Part model, mm, in its own coordinate system. A direction names the side the tool comes from. Give positions to 0.01 mm unless a question says otherwise; leave off trailing zeros. Loops run counter-clockwise (first coordinate to the right, second up) from the corner with the lowest first, then second, coordinate; pieces in that order, holes last. Notation, with made-up numbers: M 11.25,85.5 L 29.25,85.5 A30 ccw 29.25,109.5 Z; hole C 53,46 d3. An arc over 180 degrees is marked long. Answer in a Markdown table with one row per item.
from build123d import *

# Parameters (mm, degrees)
SKETCH1_W           = 83.5
SKETCH1_H           = 50
BOSS_EXTRUDE1_DEPTH = 1
SKETCH2_W           = 75
SKETCH2_H           = 15
BOSS_EXTRUDE2_DEPTH = 12.8
SKETCH3_W           = 3.3
SKETCH3_H           = 8.9
BOSS_EXTRUDE3_DEPTH = 11
BOSS_EXTRUDE4_DEPTH = 10.3
BOSS_EXTRUDE6_DEPTH = 0.5
BOSS_EXTRUDE7_DEPTH = 0.5
SKETCH7_W           = 2.9
SKETCH7_H           = 2.1
BOSS_EXTRUDE8_DEPTH = 0.8
SKETCH8_R           = 2.25
CUT_EXTRUDE1_DEPTH  = 12.2


with BuildPart() as part:
    # Sketch1 → Boss-Extrude1 (new body)
    with BuildSketch(Plane.XY):
        Rectangle(SKETCH1_W, SKETCH1_H)
    extrude(amount=BOSS_EXTRUDE1_DEPTH)

    # Sketch2 → Boss-Extrude2 (add)
    with BuildSketch(Plane.XY.offset(1)):
        with Locations((2.25, 26)):
            Rectangle(SKETCH2_W, SKETCH2_H)
    extrude(amount=BOSS_EXTRUDE2_DEPTH)



with BuildPart() as body_2:
    # Sketch3 → Boss-Extrude3 (new body)
    with BuildSketch(Plane.XY.offset(1)):
        with Locations((-45.1, -20.15)):
            Rectangle(SKETCH3_W, SKETCH3_H)
    extrude(amount=BOSS_EXTRUDE3_DEPTH)


with BuildPart() as part_1:
    add(part.part)

    add(body_2.part)  # Boss-Extrude4 merges body 2
    # Sketch4 → Boss-Extrude4 (add)
    with BuildSketch(Plane(origin=(-43.45, 0, 0), x_dir=(0, 0, -1), z_dir=(1, 0, 0))):
        with BuildLine():
            Line((-7.3, -16.2), (-1, -16.2))
            Line((-1, -16.2), (-1, -24.1))
            Line((-1, -24.1), (-7.3, -24.1))
            ThreePointArc((-7.3, -24.1), (-11.25, -20.15), (-7.3, -16.2))
        make_face()
    extrude(amount=BOSS_EXTRUDE4_DEPTH)

    # Sketch5 → Boss-Extrude6 (add)
    with BuildSketch(Plane.XZ.offset(24.1)):
        Polygon((-34.55, 7.3), (-34.55, 1), (-41.75, 1), (-43.45, 1), (-43.45, 7.3), align=None)
    extrude(amount=BOSS_EXTRUDE6_DEPTH)

    # Sketch6 → Boss-Extrude7 (add)
    with BuildSketch(Plane(origin=(0, -16.2, 0), x_dir=(1, 0, 0), z_dir=(0, 1, 0))):
        Polygon((-43.45, -7.3), (-34.55, -7.3), (-34.55, -1), (-41.75, -1), (-43.45, -1), align=None)
    extrude(amount=BOSS_EXTRUDE7_DEPTH)

    # Sketch7 → Boss-Extrude8 (add)
    with BuildSketch(Plane(origin=(-33.15, 0, 0), x_dir=(0, 0, -1), z_dir=(1, 0, 0))):
        with Locations((-2.45, -23.05)):
            Rectangle(SKETCH7_W, SKETCH7_H)
        with Locations((-2.45, -17.25)):
            Rectangle(SKETCH7_W, SKETCH7_H)
    extrude(amount=BOSS_EXTRUDE8_DEPTH)

    # Sketch8 → Cut-Extrude1 (cut)
    with BuildSketch(Plane.ZY.offset(46.75)):
        with Locations((7.3, -20.15)):
            Circle(SKETCH8_R)
    extrude(amount=-CUT_EXTRUDE1_DEPTH, mode=Mode.SUBTRACT)


solid = part_1.part
(1) Which spindle directions (+Z, -Z, +X, -X, +Y, -Y) get a long thin tool onto all of the face, cutting with end or side? Do faces 5 (the face through (-34, -16.2, 4)), 6 (the face through (-42, -24.6, 5)), 7 (the face through (2, 29, 1)), 8 (the face through (-35.25, 26, 7)), 9 (the face through (-32.35, -17, 2)). Say none if no direction does.
Recorded:
| item | result |
|---|---|
| face 5 | +Z, +X |
| face 6 | +Z, +X, -X, -Y |
| face 7 | -Z, +X, -X, +Y |
| face 8 | +Z, -X, +Y |
| face 9 | +Z, +X, -Y |
(2) Saw through at A-A (x = 31). Write the cut outline in (y, z).
Recorded:
| item | result |
|---|---|
| outline | M -25,0 L 25,0 L 25,1 L 33.5,1 L 33.5,13.8 L 18.5,13.8 L 18.5,1 L -25,1 Z |
(3) Pin check, flat tips, straight feed: pin 1 Ø5 at (y, z) = (-14.5, 9) entering from +X; pin 2 Ø2 at (x, z) = (-37, 7) entering from -Y; pin 3 Ø7 at (x, y) = (-12.5, 29) entering from -Z. Stop position of each tip, or through.
Recorded:
| item | result |
|---|---|
| pin 1 | stops at x = -33.15 |
| pin 2 | stops at y = -24.6 |
| pin 3 | stops at z = 1 |
(4) Saw through at C-C (y = 22). Write the cut outline in (x, z), plus the area to 3 significant figures.
Recorded:
| item | result |
|---|---|
| outline | M -41.75,0 L 41.75,0 L 41.75,1 L 39.75,1 L 39.75,13.8 L -35.25,13.8 L -35.25,1 L -41.75,1 Z |
| area | 1,040 mm^2 |
(5) Saw through at B-B (y = -20.15). Write the cut outline in (x, z).
Recorded:
| item | result |
|---|---|
| outline | M -46.75,1 L -41.75,1 L -41.75,0 L 41.75,0 L 41.75,1 L -33.15,1 L -33.15,11.25 L -43.45,11.25 L -43.45,12 L -46.75,12 L -46.75,9.55 L -34.55,9.55 L -34.55,5.05 L -46.75,5.05 Z |
(6) Saw through at D-D (y = -4). Write the cut outline in (x, z), plus the area to 3 significant figures.
Recorded:
| item | result |
|---|---|
| outline | M -41.75,0 L 41.75,0 L 41.75,1 L -41.75,1 Z |
| area | 83.5 mm^2 |
(7) Pull direction Y, two halves, no side cores. Call faces 1 (the face through (-34, -24.1, 4)), 2 (the face through (-40.74, -17.92, 7.01)), 3 (the face through (-45, -20, 12)), 4 (the face through (-33.15, -20, 6)): +Y half, -Y half, draft (parallel to the pull), parting line (faces both ways), or undercut.
Recorded:
| item | result |
|---|---|
| face 1 | -Y half |
| face 2 | undercut |
| face 3 | draft |
| face 4 | undercut |
(8) Drill centre lines: line 1 along Z through (x, y) = (-38, -20) (3 decimals); line 2 along Y through (x, z) = (-31, 4); line 3 along Z through (x, y) = (26.5, 11). Where is each one in solid material? Low to high.
Recorded:
| item | result |
|---|---|
| line 1 | z = 0 to 5.055, 9.545 to 11.247 |
| line 2 | y = 18.5 to 33.5 |
| line 3 | z = 0 to 1 |
